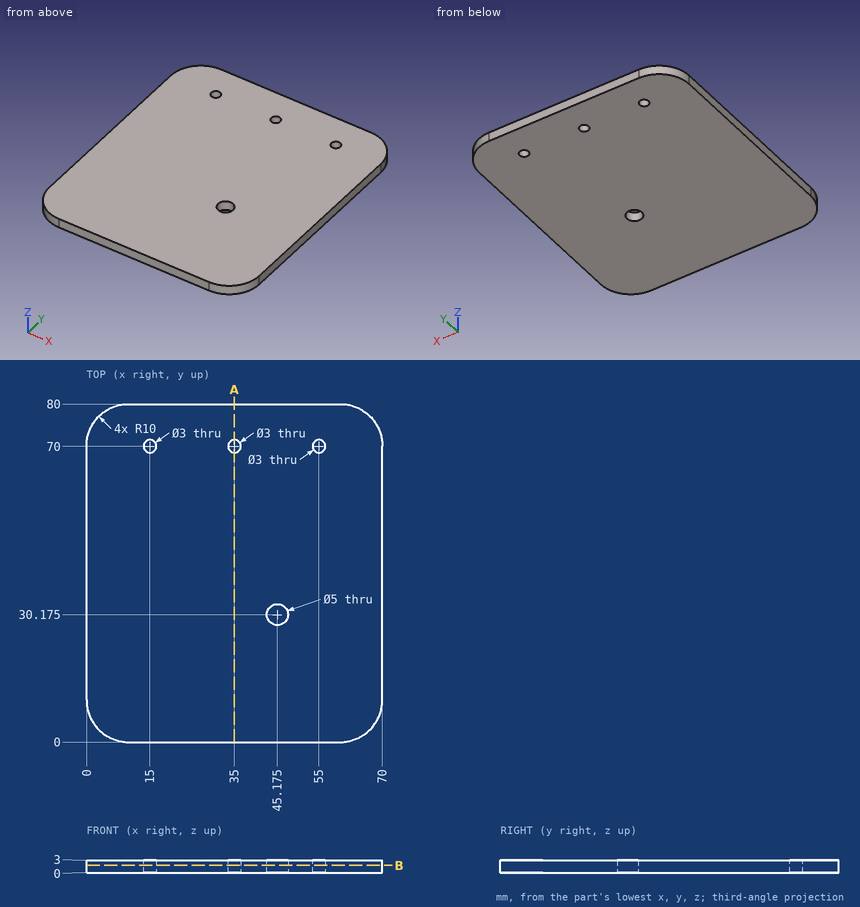
For this review, use the dimensioned drawing (mm, ordinates from the lowest corner) and the shaded views. Give positions to 0.01 mm unless a question says otherwise; leave off trailing zeros. Order: outer loops, then holes, each group sorted by start corner. A loop starts at its lowest first (then second) coordinate and runs counter-clockwise, first axis right, second up. Notation, with made-up numbers: (-10, -25) - (33, -25) arc R16 cw to (33, -7) - close; hole circle Ø5 at (89.25, 23). An arc over 180 degrees is marked (long way). Use CSV: the item, a comma, the result in double quotes. Start each with the question number.
Q1. To check wall thickness, follow line 1 along X through (y, z) = (70, 2.45); line 2 along Y through (x, z) = (35, 1.8); line 3 along Y through (x, z) = (14.5, 1.25). State the ranges of each line that lie inside material, in increasing order. Write a range as [from, to].
Q2. We need section B-B, the plane z = 1.75. Write out the cut boundary in (x, y) (3 decimals).
Q3. Clearance check with a flat-ended pin moving along its axis: pin 1 Ø2.5 at (x, y) = (15, 70) entering from -Z. State where the tip first meets the part, or that it passes through.
Q4. We need section A-A, the plane x = 35. Write out the cut boundary in (y, z), and give its area (3 significant figures).
Outcome:
1,line 1,"x = [0, 13.5], [16.5, 33.5], [36.5, 53.5], [56.5, 70]"
1,line 2,"y = [0, 68.5], [71.5, 80]"
1,line 3,"y = [0, 68.59], [71.41, 80]"
2,outline,"(0, 10) arc R10 ccw to (10, 0) - (60, 0) arc R10 ccw to (70, 10) - (70, 70) arc R10 ccw to (60, 80) - (10, 80) arc R10 ccw to (0, 70) - close; hole circle Ø3 at (15, 70); hole circle Ø3 at (35, 70); hole circle Ø5 at (45.175, 30.175); hole circle Ø3 at (55, 70)"
3,pin 1,"passes through"
4,outline,"(0, 0) - (68.5, 0) - (68.5, 3) - (0, 3) - close; (71.5, 0) - (80, 0) - (80, 3) - (71.5, 3) - close"
4,area,"231 mm^2"
